from build123d import *

# Parameters (mm, degrees)
BOSS_EXTRUDE1_DEPTH                 = 228.6
BOSS_EXTRUDE1_DEPTH_BACK            = 228.6
SKETCH3_R                           = 6.35
CHAMFER1_SIZE                       = 0.254
M6X1_0_TAPPED_HOLE1_D               = 5
M6X1_0_TAPPED_HOLE1_DEPTH           = 25
M6X1_0_TAPPED_HOLE1_TIP             = 1.502151548
M6X1_0_TAPPED_HOLE1_ON_FACE_2_D     = 5
M6X1_0_TAPPED_HOLE1_ON_FACE_2_DEPTH = 25
M6X1_0_TAPPED_HOLE1_ON_FACE_2_TIP   = 1.502151548


with BuildPart() as part:
    # Sketch3 → Boss-Extrude1 (new, two sides: drawn at the far end of the back side and taken through both)
    with BuildSketch(Plane.XY.offset(-BOSS_EXTRUDE1_DEPTH_BACK)):
        Circle(SKETCH3_R)
    extrude(amount=BOSS_EXTRUDE1_DEPTH + BOSS_EXTRUDE1_DEPTH_BACK)

    # Chamfer1
    chamfer1_edges = [part.edges().sort_by_distance(p)[0] for p in [
        (-6.35, 0, -228.6),
        (-6.35, 0, 228.6),
    ]]
    chamfer(chamfer1_edges, length=CHAMFER1_SIZE)

    # M6x1.0 Tapped Hole1
    with Locations(Plane(origin=(0, 0, -228.6), x_dir=(-1, 0, 0), z_dir=(0, 0, -1))):
        with Locations((0, 0)):
            Hole(M6X1_0_TAPPED_HOLE1_D / 2, depth=M6X1_0_TAPPED_HOLE1_DEPTH)
            with Locations((0, 0, -(M6X1_0_TAPPED_HOLE1_DEPTH + M6X1_0_TAPPED_HOLE1_TIP / 2))):  # 118° drill point
                Cone(0, M6X1_0_TAPPED_HOLE1_D / 2, M6X1_0_TAPPED_HOLE1_TIP, mode=Mode.SUBTRACT)

    # M6x1.0 Tapped Hole1 on face 2
    with Locations(Plane.XY.offset(228.6)):
        with Locations((0, 0)):
            Hole(M6X1_0_TAPPED_HOLE1_ON_FACE_2_D / 2, depth=M6X1_0_TAPPED_HOLE1_ON_FACE_2_DEPTH)
            with Locations((0, 0, -(M6X1_0_TAPPED_HOLE1_ON_FACE_2_DEPTH + M6X1_0_TAPPED_HOLE1_ON_FACE_2_TIP / 2))):  # 118° drill point
                Cone(0, M6X1_0_TAPPED_HOLE1_ON_FACE_2_D / 2, M6X1_0_TAPPED_HOLE1_ON_FACE_2_TIP, mode=Mode.SUBTRACT)


solid = part.part
Geometry: final body of the model. Coordinates: model frame, mm. Give positions to 0.01 mm unless a question says otherwise; leave off trailing zeros. Order: outer loops, then holes, each group sorted by start corner. A loop starts at its lowest first (then second) coordinate and runs counter-clockwise, first axis right, second up. Notation, with made-up numbers: (-24.5, 46.25) -> (33.5, 46.25) arc R31 cw to (33.5, 73.25) -> close; hole circle Ø4 at (-26, 85.25). An arc over 180 degrees is marked (long way). Put each result on its own line as item: value.
Q1. Section A-A, the plane z = -177. Return loops of the section in (x, y).
Here are the results:
outline: circle Ø12.7 at (0, 0)
Q2. Material intervals for L1, parallel to Y at x = 0, z = -210; L2, parallel to Y at x = 1.5, z = 121; L3, parallel to X at y = 5.75, z = 122, sorted ascending.
Here are the results:
L1: y = -6.35 to -2.5, 2.5 to 6.35
L2: y = -6.17 to 6.17
L3: x = -2.69 to 2.69
Q3. Pin query (flat end, axial travel): pin 1 (1.5 mm diameter, centred on y = 3, z = -53, fed in from +X); pin 2 (6 mm diameter, centred on y = -5, z = -68, fed in from -X); pin 3 (3 mm diameter, centred on x = 0, y = 0, fed in from -Z). Return the tip coordinate at first contact, or that it passes through.
Here are the results:
pin 1: stops at x = 5.94
pin 2: stops at x = -6.03
pin 3: stops at z = -203
